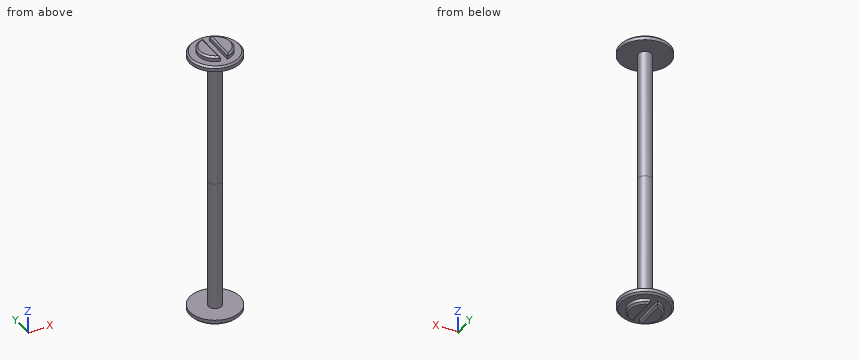
```python
from build123d import *

# Parameters (mm, degrees)
SKETCH1_R           = 7.5
BOSS_EXTRUDE1_DEPTH = 1.5
SKETCH2_R           = 5
BOSS_EXTRUDE2_DEPTH = 1.5
SKETCH3_R           = 2
BOSS_EXTRUDE3_DEPTH = 39
SKETCH4_W           = 2
SKETCH4_H           = 12
CUT_EXTRUDE1_DEPTH  = 1.5
CHAMFER1_SIZE       = 0.5


with BuildPart() as part:
    # Sketch1 → Boss-Extrude1 (new body)
    with BuildSketch(Plane.XY):
        Circle(SKETCH1_R)
    extrude(amount=BOSS_EXTRUDE1_DEPTH)

    # Sketch2 → Boss-Extrude2 (add)
    with BuildSketch(Plane.XY.offset(1.5)):
        Circle(SKETCH2_R)
    extrude(amount=BOSS_EXTRUDE2_DEPTH)

    # Sketch3 → Boss-Extrude3 (add)
    with BuildSketch(Plane(origin=(0, 0, 0), x_dir=(-1, 0, 0), z_dir=(0, 0, -1))):
        Circle(SKETCH3_R)
    extrude(amount=BOSS_EXTRUDE3_DEPTH)

    # Sketch4 → Cut-Extrude1 (cut)
    with BuildSketch(Plane.XY.offset(3)):
        Rectangle(SKETCH4_W, SKETCH4_H)
    extrude(amount=-CUT_EXTRUDE1_DEPTH, mode=Mode.SUBTRACT)

    # Mirror1: part across plane


with BuildPart() as part_1:
    add(part.part)
    add(part.part.mirror(Plane(origin=(0, 0, -39), x_dir=(1, 0, 0), z_dir=(0, 0, -1))))

    # Chamfer1
    chamfer1_edges = [part_1.edges().sort_by_distance(p)[0] for p in [
        (-5, 0, 3),
        (5, 0, 3),
        (-1, 0, 3),
        (1, 0, 3),
        (-7.5, 0, 1.5),
        (5, 0, -81),
        (1, 0, -81),
        (-7.5, 0, -79.5),
        (-5, 0, -81),
        (-1, 0, -81),
    ]]
    chamfer(chamfer1_edges, length=CHAMFER1_SIZE)


solid = part_1.part
```
Part model, mm, in its own coordinate system. Round coordinates to 2 decimals unless told otherwise and drop trailing zeros. Loops run counter-clockwise (first coordinate to the right, second up) from the corner with the lowest first, then second, coordinate; pieces in that order, holes last.
Item 1: Drop flat-ended pins along their axis: P1, Ø8, axis at y = 0, z = -16.5, coming from the +X side; P2, Ø1, axis at y = -2, z = -65.5, coming from the +X side; P3, Ø5, axis at x = 3.5, z = -57, coming from the +Y side. Give the stop position or say it passes through.
Item 2: Cut at A-A, the plane x = 0. Give the cut face in (y, z).
Item 3: Cut at B-B, the plane z = -57.5. Give the cut face in (x, y), then the cut area to 3 significant figures.
Item 4: Drill centre lines: line 1 (Z direction, x = 6, y = -3.25); line 2 (Z direction, x = -4, y = -2); line 3 (Y direction, x = 0.25, z = -34.5). Where is each one in solid material? Low to high.
A:
1. P1: stops at x = 2
1. P2: stops at x = 1.32
1. P3: stops at y = 1.73
2. outline: (-7.5, -79) - (-7, -79.5) - (7, -79.5) - (7.5, -79) - (7.5, -78) - (2, -78) - (2, 0) - (7.5, 0) - (7.5, 1) - (7, 1.5) - (-7, 1.5) - (-7.5, 1) - (-7.5, 0) - (-2, 0) - (-2, -78) - (-7.5, -78) - close
3. outline: circle Ø4 at (0, 0)
3. area: 12.6 mm2
4. line 1: z = -79.5 to -78, 0 to 1.5
4. line 2: z = -81 to -78, 0 to 3
4. line 3: y = -1.98 to 1.98
